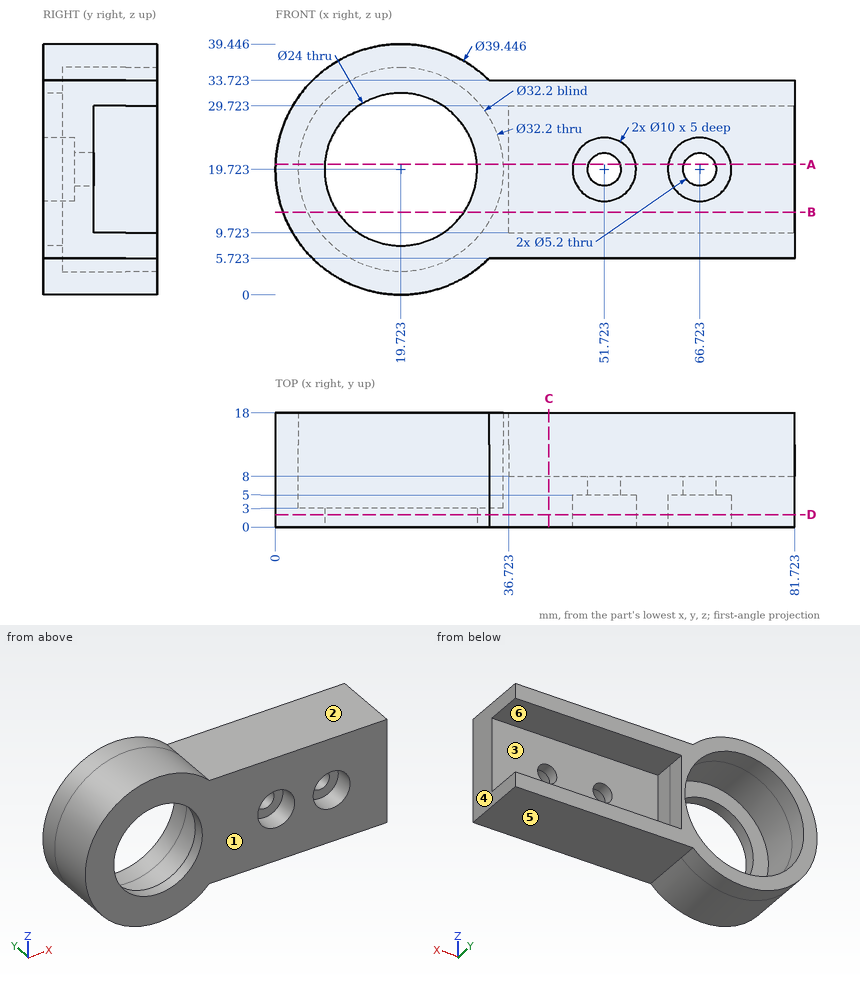
Could you check a few things on this drawing? It's one solid part, dimensions in mm from its lowest x, y, z. A direction names the side the tool comes from. Coordinates: 2 decimals unless noted, no trailing zeros. Order: outer loops, then holes, each group sorted by start corner. A loop starts at its lowest first (then second) coordinate and runs counter-clockwise, first axis right, second up. Notation, with made-up numbers: M -28.75,56 L 10.25,56 A28 cw 10.25,85 Z; hole C -22.75,67.5 d4. An arc over 180 degrees is marked long. Use a Markdown table: item, result. Add a question column.
Q1. We'd pull the mould along Z, two halves only. Please class the marked faces 1, 2 and 3: pulls with the +Z half, pulls with the -Z half, needs draft (parallel to the pull), parting line crosses it, or undercut.
Q2. If I drill on L1, parallel to Z at x = 66, y = 12; L2, parallel to Z at x = 42, y = 6.5; L3, parallel to Y at x = 51, z = 13, over which ranges is the centre line in solid material (lowest first)?
Q3. I want a section at B-B on z = 13. List the corners of the cut face in (x, y) for me.
Q4. I want a section at A-A on z = 20.5. Give the number of separate pieces and of enclosed holes in the cut face, then the cut area to 3 significant figures.
Q5. I want a section at D-D on y = 2. List the corners of the cut face in (x, z) for me.
Q6. I'm going to push flat-ended pins straight in: pin 1 (1.5 mm diameter, centred on y = 15.5, z = 18.5, fed in from +X); pin 2 (10 mm diameter, centred on x = 67.5, y = 2, fed in from -Z); pin 3 (8 mm diameter, centred on x = 51.72, z = 19.72, fed in from -Y). Where does each tip first touch, or does it pass through?
Q7. Which directions (+Z, -Z, +X, -X, +Y, -Y) give clear straight access to the entire face, cutting with the end or side of a thin tool? Please do the marked faces 4, 5 and 6.
Q8. I want a section at C-C on x = 43. List the corners of the cut face in (y, z) for me, then the cut area to 3 significant figures.
Checked values:
| question | item | result |
|---|---|---|
| 1 | face 1 | needs draft |
| 1 | face 2 | pulls with the +Z half |
| 1 | face 3 | undercut |
| 2 | L1 | 5.72 to 9.72, 29.72 to 33.72 |
| 2 | L2 | 5.72 to 33.72 |
| 2 | L3 | 0 to 8 |
| 3 | outline | M 1.18,0 L 9.78,0 L 9.78,3 L 5.09,3 L 5.09,18 L 1.18,18 Z; M 29.66,0 L 81.72,0 L 81.72,8 L 36.72,8 L 36.72,18 L 34.35,18 L 34.35,3 L 29.66,3 Z |
| 4 | separate pieces | 4 |
| 4 | enclosed holes | 0 |
| 4 | area | 338 mm² |
| 5 | outline | M 33.62,5.72 L 81.72,5.72 L 81.72,33.72 L 33.62,33.72 A19.72 ccw long Z; hole C 19.72,19.72 d24; hole C 51.72,19.72 d10; hole C 66.72,19.72 d10 |
| 6 | pin 1 | x = 36.72 |
| 6 | pin 2 | z = 5.72 |
| 6 | pin 3 | y = 5 |
| 7 | face 4 | +Z, -Z, +X, +Y, -Y |
| 7 | face 5 | -Z, +X, +Y, -Y |
| 7 | face 6 | +X, +Y |
| 8 | outline | M 0,5.72 L 18,5.72 L 18,9.72 L 8,9.72 L 8,29.72 L 18,29.72 L 18,33.72 L 0,33.72 Z |
| 8 | area | 304 mm² |
